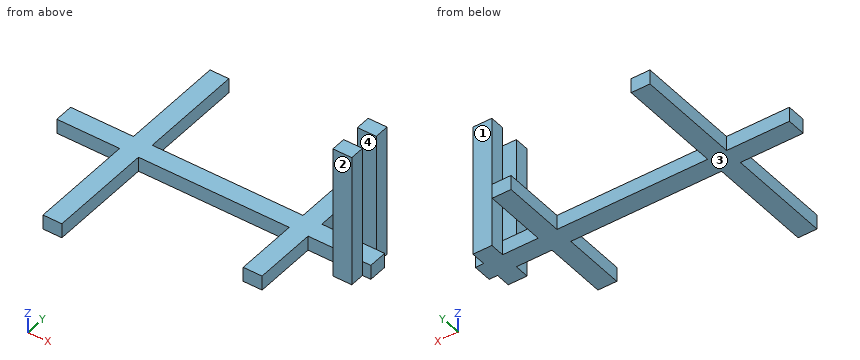
from build123d import *

# Parameters (mm, degrees)
F0_W          = 750
F0_H          = 35
F1_DEPTH      = 22.5
F2_W          = 45
F2_H          = 150
F2_H_2        = 250
F3_DEPTH      = 17.5
F4_W          = 45
F4_H          = 35
F5_DEPTH      = 300
F5_DEPTH_BACK = 17.5


with BuildPart() as f1:
    # F0 (on Front) → F1 (new body, symmetric)
    with BuildSketch(Plane.XZ):
        Rectangle(F0_W, F0_H)
    extrude(amount=F1_DEPTH, both=True)

    # F2 (on Top) → F3 (join, symmetric)
    with BuildSketch(Plane.XY):
        with Locations((202.5, 97.5)):
            Rectangle(F2_W, F2_H)
        with Locations((202.5, -97.5)):
            Rectangle(F2_W, F2_H)
        with Locations((-202.5, 147.5)):
            Rectangle(F2_W, F2_H_2)
        with Locations((-202.5, -147.5)):
            Rectangle(F2_W, F2_H_2)
    extrude(amount=F3_DEPTH, both=True)

    # F4 (on Top) → F5 (join, two sides)
    with BuildSketch(Plane.XY) as f5_sk:
        with Locations((332.5, 40)):
            Rectangle(F4_W, F4_H)
        with Locations((332.5, -40)):
            Rectangle(F4_W, F4_H)
    extrude(amount=F5_DEPTH)
    extrude(f5_sk.sketch, amount=-F5_DEPTH_BACK)


solid = f1.part
Can you work these out from the model? Positions are in its coordinate system, mm. Face numbers are marked on the shaded views. Round coordinates to 2 decimals unless told otherwise and drop trailing zeros. Write each loop counter-clockwise with the first axis right and the second up, starting at its lowest first coordinate (ties: lowest second). Pieces come first, ordered by that corner, then holes. Notation, with made-up numbers: (60.25, 35.5) -> (69.25, 35.5) arc R32 ccw to (69.25, 65.5) -> close; hole circle Ø3 at (7.5, -33). An arc over 180 degrees is marked (long way). One line per question, with ' | ' between items. Start each with the question number.
1) Suppose I cut it at C-C on z = 4.5. Write out the boundary of the cut face in (x, y), then the cut area to 3 significant figures.
2) Suppose I cut it at A-A on y = 109.5. Write out the boundary of the cut face in (x, z).
3) If we mould it in two halves opening along Y, with no side actions, what happens to the marked faces 1, 2, 3 and 4? For each: released by +Y, released by -Y, zero draft, split by the parting line, or undercut.
4) Suppose I cut it at B-B on z = 166. Write out the boundary of the cut face in (x, y).
5) Suppose I cut it at D-D on x = 32.5. Write out the boundary of the cut face in (y, z), then the cut area to 4 significant figures.
6) I need wall thicknesses on line 1 (X direction, y = 27, z = 269); line 2 (Y direction, x = 338, z = 40); line 3 (Z direction, x = 207.5, y = -39). Which ranges of each line are inside material? Lowest first, please. Write a range as [from, to].
7) I'm going to push flat-ended pins straight in: P1, Ø16, axis at x = 361.5, z = 3, coming from the -Y side; P2, Ø17.5, axis at y = -192, z = -5.5, coming from the -X side; P3, Ø17.5, axis at y = -144.5, z = -7.5, coming from the +X side. Where does each tip first touch, or does it pass through?
Return value:
1) outline: (-375, -22.5) -> (-225, -22.5) -> (-225, -272.5) -> (-180, -272.5) -> (-180, -22.5) -> (180, -22.5) -> (180, -172.5) -> (225, -172.5) -> (225, -22.5) -> (310, -22.5) -> (310, -57.5) -> (355, -57.5) -> (355, -22.5) -> (375, -22.5) -> (375, 22.5) -> (355, 22.5) -> (355, 57.5) -> (310, 57.5) -> (310, 22.5) -> (225, 22.5) -> (225, 172.5) -> (180, 172.5) -> (180, 22.5) -> (-180, 22.5) -> (-180, 272.5) -> (-225, 272.5) -> (-225, 22.5) -> (-375, 22.5) -> close | area: 72,900 mm2
2) outline: (-225, -17.5) -> (-180, -17.5) -> (-180, 17.5) -> (-225, 17.5) -> close; (180, -17.5) -> (225, -17.5) -> (225, 17.5) -> (180, 17.5) -> close
3) face 1: released by +Y | face 2: released by -Y | face 3: zero draft | face 4: undercut
4) outline: (310, -57.5) -> (355, -57.5) -> (355, -22.5) -> (310, -22.5) -> close; (310, 22.5) -> (355, 22.5) -> (355, 57.5) -> (310, 57.5) -> close
5) outline: (-22.5, -17.5) -> (22.5, -17.5) -> (22.5, 17.5) -> (-22.5, 17.5) -> close | area: 1,575 mm2
6) line 1: x = [310, 355] | line 2: y = [-57.5, -22.5], [22.5, 57.5] | line 3: z = [-17.5, 17.5]
7) P1: stops at y = -57.5 | P2: stops at x = -225 | P3: stops at x = 225
